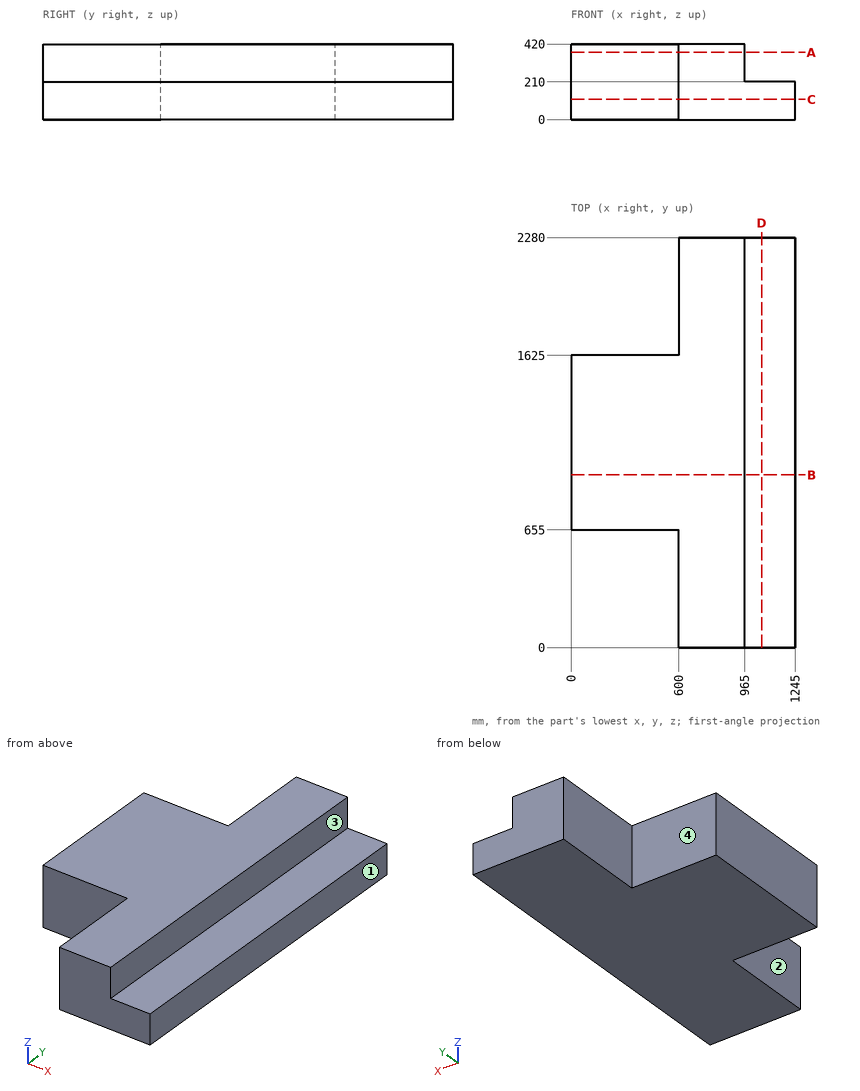
Can you work these out from the drawing? Everything is in mm from the part's minimum corner. A direction names the side the tool comes from. Round coordinates to 2 decimals unless told otherwise and drop trailing zeros. Order: outer loops, then holes, each group sorted by start corner. A loop starts at its lowest first (then second) coordinate and runs counter-clockwise, first axis right, second up.
(1) If we section it at C-C (z = 112): Please give me the cut outline in (x, y).
Results are:
outline: (0, 655) - (600, 655) - (600, 0) - (1245, 0) - (1245, 2280) - (600, 2280) - (600, 1625) - (0, 1625) - close
(2) On a 3-axis mill with a long thin cutter (end or side, diameter ignored), from which of +Z, -Z, +X, -X, +Y, -Y can I reach the whole of each face in a straight line? I mean the marked faces 1, 2, 3 and 4. Say none if no direction works.
Results are:
face 1: +Z, -Z, +X, +Y, -Y
face 2: +Z, -Z, -X, -Y
face 3: +Z, +X, +Y, -Y
face 4: +Z, -Z, -X, +Y
(3) If we section it at B-B (y = 961): Please give me the cut outline in (x, z), plus the area to 3 significant figures.
Results are:
outline: (0, 0) - (1245, 0) - (1245, 210) - (965, 210) - (965, 420) - (0, 420) - close
area: 464,000 mm2
(4) If I drill on L1, parallel to Y at x = 214.5, z = 126.5; L2, parallel to X at y = 208.5, z = 306; L3, parallel to X at y = 472, z = 148.5, over which ranges is the centre line in solid material (lowest first)?
Results are:
L1: y = 655 to 1625
L2: x = 600 to 965
L3: x = 600 to 1245
(5) If we section it at D-D (x = 1059): Please give me the cut outline in (y, z).
Results are:
outline: (0, 0) - (2280, 0) - (2280, 210) - (0, 210) - close
(6) If we section it at A-A (z = 373.5): Please give me the cut outline in (x, y), plus the area to 3 significant figures.
Results are:
outline: (0, 655) - (600, 655) - (600, 0) - (965, 0) - (965, 2280) - (600, 2280) - (600, 1625) - (0, 1625) - close
area: 1,410,000 mm2
(7) I'm going to push flat-ended pins straight in: pin 1 (4 mm diameter, centred on y = 376, z = 330, fed in from +X); pin 2 (4 mm diameter, centred on x = 303.5, z = 301.5, fed in from +Y); pin 3 (12 mm diameter, centred on y = 421, z = 74, fed in from -X); pin 4 (2 mm diameter, centred on x = 870, y = 1163.5, fed in from -Z). Where does each tip first touch, or does it pass through?
Results are:
pin 1: stops at x = 965
pin 2: stops at y = 1625
pin 3: stops at x = 600
pin 4: stops at z = 0
